Geometry: final body of the model. Coordinates: model frame, mm. A direction names the side the tool comes from. Give positions to 0.01 mm unless a question says otherwise; leave off trailing zeros. Write each loop counter-clockwise with the first axis right and the second up, starting at its lowest first coordinate (ties: lowest second). Pieces come first, ordered by that corner, then holes. Notation, with made-up numbers: (78, 85) - (136, 85) arc R27 cw to (136, 122) - close; hole circle Ø9 at (59.5, 5). An arc over 180 degrees is marked (long way). Return JSON: item names as keys, results as strings.
from build123d import *

# Parameters (mm, degrees)
F1_DEPTH  = 426
F3_DEPTH  = 4
F4_R      = 2
F7_DEPTH  = 4
F10_DEPTH = 4


# Not quite as in the source:
# - a feature names something its author has since deleted; it is built from what else it names


with BuildPart() as f1:
    # F0 (on Top) → F1 (new body)
    with BuildSketch(Plane.XY):
        Polygon((495, 0), (0, 0), (0, -343), (200, -343), (200, -1261), (204, -1261), (204, -339), (4, -339), (4, -4), (491, -4), (491, -1261), (495, -1261), align=None)
    extrude(amount=F1_DEPTH)

    # F2 (on Top) → F3 (join)
    with BuildSketch(Plane.XY):
        Polygon((0, -343), (200, -343), (200, -1261), (495, -1261), (495, 0), (0, 0), align=None)
    extrude(amount=-F3_DEPTH)

    # F4
    f4_edges = [f1.edges().sort_by_distance(p)[0] for p in [
        (100, -343, -4),
        (0, -171.5, -4),
        (247.5, 0, -4),
        (200, -343, 211),
        (0, -343, 211),
        (0, 0, 211),
        (495, 0, 211),
        (200, -802, -4),
        (495, -630.5, -4),
    ]]
    fillet(f4_edges, radius=F4_R)

    # F6 (on offset) → F7 (join)
    with BuildSketch(Plane.XZ.offset(961)):
        Polygon((269, 0), (491, 0), (491, 355), align=None)
    extrude(amount=F7_DEPTH)

    # F9 (on offset) → F10 (join)
    with BuildSketch(Plane.XZ.offset(361)):
        Polygon((204, 355), (204, 0), (426, 0), align=None)
    extrude(amount=F10_DEPTH)


solid = f1.part
Q1. Section query D-D, the plane z = 157.5. Return the cut outline in (x, y).
Answer key:
{"outline": "(0, -341) arc R2 ccw to (2, -343) - (198, -343) arc R2 cw to (200, -345) - (200, -1261) - (204, -1261) - (204, -365) - (327.51, -365) - (327.51, -361) - (204, -361) - (204, -339) - (4, -339) - (4, -4) - (491, -4) - (491, -961) - (367.49, -961) - (367.49, -965) - (491, -965) - (491, -1261) - (495, -1261) - (495, -2) arc R2 ccw to (493, 0) - (2, 0) arc R2 ccw to (0, -2) - close"}
Q2. Section query C-C, the plane z = 270. Return the cut outline in (x, y), plus the area to 3 significant figures.
Answer key:
{"outline": "(0, -341) arc R2 ccw to (2, -343) - (198, -343) arc R2 cw to (200, -345) - (200, -1261) - (204, -1261) - (204, -365) - (257.15, -365) - (257.15, -361) - (204, -361) - (204, -339) - (4, -339) - (4, -4) - (491, -4) - (491, -961) - (437.85, -961) - (437.85, -965) - (491, -965) - (491, -1261) - (495, -1261) - (495, -2) arc R2 ccw to (493, 0) - (2, 0) arc R2 ccw to (0, -2) - close", "area": "13,300 mm^2"}
Q3. Mould query, pull axis Y, two halves, no side actions, for faces 4 (the flat face through (251, 0, 215)), 5 (the flat face through (299, -483, -4)), 6 (the flat face through (316.55, -362.97, 175.02)). Classes: pulls with the +Y half, pulls with the -Y half, needs draft (parallel to the pull), parting line crosses it, or undercut.
Answer key:
{"face 4": "pulls with the +Y half", "face 5": "needs draft", "face 6": "undercut"}
Q4. Section query B-B, the plane y = -777. Return the cut outline in (x, z).
Answer key:
{"outline": "(200, -2) arc R2 ccw to (202, -4) - (493, -4) arc R2 ccw to (495, -2) - (495, 426) - (491, 426) - (491, 0) - (204, 0) - (204, 426) - (200, 426) - close"}
Q5. Section query A-A, the plane x = 147. Return the cut outline in (y, z), plus the area to 3 significant figures.
Answer key:
{"outline": "(-343, -2) arc R2 ccw to (-341, -4) - (-2, -4) arc R2 ccw to (0, -2) - (0, 426) - (-4, 426) - (-4, 0) - (-339, 0) - (-339, 426) - (-343, 426) - close", "area": "4,780 mm^2"}
Q6. Pin query (flat end, axial travel): P1, Ø1, axis at y = -372, z = 280.5, coming from the -X side; P2, Ø1, axis at x = 284.5, y = -625.5, coming from the +Z side; P3, Ø12, axis at x = 114, z = 226.5, coming from the -Y side. Return the tip coordinate at first contact, or that it passes through.
Answer key:
{"P1": "stops at x = 200", "P2": "stops at z = 0", "P3": "stops at y = -343"}
Q7. Set-up query: faces 1 (the flat face through (428, -961, 101)), 2 (the flat face through (200, -797, 215)), 3 (the flat face through (428, -965, 101)). Return all of +Z, -Z, +X, -X, +Y, -Y with unobstructed straight access to the full face (end or side cutting, diameter ignored); none if empty.
Answer key:
{"face 1": "+Z", "face 2": "+Z, -Z, -X, -Y", "face 3": "+Z, -Y"}
Q8. Material intervals for probe 1 along Y at (x, z) = (350.5, 27); probe 2 along Y at (x, z) = (291, 98); probe 3 along X at (y, z) = (-1098, 125.5), sorted ascending. Write a range as [from, to].
Answer key:
{"probe 1": "y = [-965, -961], [-365, -361], [-4, 0]", "probe 2": "y = [-365, -361], [-4, 0]", "probe 3": "x = [200, 204], [491, 495]"}
